Part model, mm, in its own coordinate system. A direction names the side the tool comes from. Coordinates: 2 decimals unless noted, no trailing zeros. Order: outer loops, then holes, each group sorted by start corner. A loop starts at its lowest first (then second) coordinate and runs counter-clockwise, first axis right, second up. Notation, with made-up numbers: M 52.25,-38.75 L 60.25,-38.75 A27 cw 60.25,0.25 Z; hole C 54.5,73 d10. An arc over 180 degrees is marked long. Write item = value, one per line. Start each with the question number.
from build123d import *

# Parameters (mm, degrees)
SKETCH_1_R          = 1.5
SKETCH_1_R_2        = 45
EXTRUDE_1_DEPTH     = 3
SKETCH_2_R          = 34
SKETCH_2_R_2        = 2
CUT_EXTRUDE_1_DEPTH = 157.95222203
SKETCH_3_W          = 10
SKETCH_3_H          = 3
EXTRUDE_2_DEPTH     = 2.5
SKETCH_5_R          = 0.75
CUT_EXTRUDE_2_DEPTH = 157.95222203
SKETCH_8_R          = 0.9
CUT_EXTRUDE_3_DEPTH = 157.95222203


with BuildPart() as part:
    # 草图1 → Extrude 1 (new body)
    with BuildSketch(Plane(origin=(0, 0, 0), x_dir=(1, 0, 0), z_dir=(0, 1, 0))):
        with BuildLine():
            Line((-60, 24.852813742), (-60, -24.852813742))
            Line((-60, -24.852813742), (-24.852813742, -60))
            Line((-24.852813742, -60), (24.852813742, -60))
            Line((24.852813742, -60), (60, -24.852813742))
            Line((60, -24.852813742), (60, 24.852813742))
            Line((60, 24.852813742), (60, 45.147186258))
            Line((60, 45.147186258), (44.671002135, 128.6127102))
            ThreePointArc((44.671002135, 128.6127102), (37.801285013, 140.366427757), (25, 145))
            Line((25, 145), (-25, 145))
            ThreePointArc((-25, 145), (-37.801285013, 140.366427757), (-44.671002135, 128.6127102))
            Line((-44.671002135, 128.6127102), (-60, 45.147186258))
            Line((-60, 45.147186258), (-60, 24.852813742))
        make_face()
        with Locations(Location((-6.35, 52, 0), (0, 0, 270))):
            Circle(SKETCH_1_R, mode=Mode.SUBTRACT)
        with Locations(Location((6.35, 52, 0), (0, 0, 270))):
            Circle(SKETCH_1_R, mode=Mode.SUBTRACT)
        with Locations(Location((6.35, -52, 0), (0, 0, 90))):
            Circle(SKETCH_1_R, mode=Mode.SUBTRACT)
        with Locations(Location((-6.35, -52, 0), (0, 0, 90))):
            Circle(SKETCH_1_R, mode=Mode.SUBTRACT)
        with Locations(Location((0, 0, 0), (0, 0, 270))):
            Circle(SKETCH_1_R_2, mode=Mode.SUBTRACT)
    extrude(amount=EXTRUDE_1_DEPTH)

    # 草图2 → 切除-拉伸1 (cut, through all)
    with BuildSketch(Plane(origin=(0, 3, 0), x_dir=(1, 0, 0), z_dir=(0, 1, 0))):
        with Locations(Location((0, 105, 0), (0, 0, 270))):
            Circle(SKETCH_2_R)
        with Locations(Location((-35, 52.5, 0), (0, 0, 270))):
            Circle(SKETCH_2_R_2)
        with Locations(Location((35, 52.5, 0), (0, 0, 270))):
            Circle(SKETCH_2_R_2)
        with Locations(Location((40.783850417, 124.017821778, 0), (0, 0, 270))):
            Circle(SKETCH_2_R_2)
        with Locations(Location((-40.783850417, 124.017821778, 0), (0, 0, 90))):
            Circle(SKETCH_2_R_2)
        with Locations(Location((-50, 40.147186258, 0), (0, 0, 270))):
            Circle(SKETCH_2_R_2)
        with Locations(Location((50, 40.147186258, 0), (0, 0, 90))):
            Circle(SKETCH_2_R_2)
        Polygon((28.087242696, 35.158310508), (35.158310508, 28.087242696), (44.547727215, 37.476659403), (37.476659403, 44.547727215), align=None)
        Polygon((-37.476659403, 44.547727215), (-44.547727215, 37.476659403), (-35.158310508, 28.087242696), (-28.087242696, 35.158310508), align=None)
    extrude(amount=-CUT_EXTRUDE_1_DEPTH, mode=Mode.SUBTRACT)

    # 草图3 → 凸台-拉伸2 (add)
    with BuildSketch(Plane.XY.offset(60)):
        with Locations((-12.5, 1.5)):
            Rectangle(SKETCH_3_W, SKETCH_3_H)
        with Locations((12.5, 1.5)):
            Rectangle(SKETCH_3_W, SKETCH_3_H)
    extrude(amount=EXTRUDE_2_DEPTH)

    # 草图5 → 切除-拉伸2 (cut, through all)
    with BuildSketch(Plane(origin=(0, 3, 0), x_dir=(1, 0, 0), z_dir=(0, 1, 0))):
        with Locations((-18.25, -60)):
            Circle(SKETCH_5_R)
        with Locations((-6.75, -60)):
            Circle(SKETCH_5_R)
        with Locations((6.75, -60)):
            Circle(SKETCH_5_R)
        with Locations((18.25, -60)):
            Circle(SKETCH_5_R)
        Polygon((-44.794179278, 105.501282313), (-40.264845988, 88.597580353), (-38.332994336, 89.115218444), (-42.862327625, 106.018920404), align=None)
        Polygon((42.862327625, 106.018920404), (38.332994336, 89.115218444), (40.264845988, 88.597580353), (44.794179278, 105.501282313), align=None)
        with BuildLine():
            Line((-60, 0), (-60, -24.852813742))
            Line((-60, -24.852813742), (-42.426406871, -42.426406871))
            ThreePointArc((-42.426406871, -42.426406871), (-55.432771951, -22.961005942), (-60, 0))
        make_face()
        with BuildLine():
            Line((60, -24.852813742), (42.426406871, -42.426406871))
            ThreePointArc((42.426406871, -42.426406871), (55.432771951, -22.961005942), (60, 0))
            Line((60, 0), (60, -24.852813742))
        make_face()
    extrude(amount=-CUT_EXTRUDE_2_DEPTH, mode=Mode.SUBTRACT)

    # 草图8 → 切除-拉伸3 (cut, through all)
    with BuildSketch(Plane(origin=(0, 3, 0), x_dir=(1, 0, 0), z_dir=(0, 1, 0))):
        with Locations((-44.561242137, 104.63194907)):
            Circle(SKETCH_8_R)
        with Locations((-42.629390484, 105.14958716)):
            Circle(SKETCH_8_R)
        with Locations((-38.565931476, 89.984551687)):
            Circle(SKETCH_8_R)
        with Locations((-40.497783129, 89.466913597)):
            Circle(SKETCH_8_R)
        with Locations((40.497783129, 89.466913597)):
            Circle(SKETCH_8_R)
        with Locations((38.565931476, 89.984551687)):
            Circle(SKETCH_8_R)
        with Locations((42.629390484, 105.14958716)):
            Circle(SKETCH_8_R)
        with Locations((44.561242137, 104.63194907)):
            Circle(SKETCH_8_R)
    extrude(amount=-CUT_EXTRUDE_3_DEPTH, mode=Mode.SUBTRACT)


solid = part.part
Item 1: Cut at A-A, the plane x = 0. Write the cut outline in (y, z), and give its area (3 significant figures).
Item 2: Cut at C-C, the plane z = -31.5. Write the cut outline in (x, y).
Item 3: Flat gauge pins, fed straight in: pin 1 (4 mm diameter, centred on x = -6.35, z = -52, fed in from -Y); pin 2 (1.2 mm diameter, centred on y = 2, z = 61.5, fed in from +X); pin 3 (0.9 mm diameter, centred on x = -21.5, y = 1, fed in from +Z); pin 4 (1.5 mm diameter, centred on x = -29, y = 1.5, fed in from -Z). Where does each tip first touch, or does it go through?
Item 4: Cut at B-B, the plane z = 21. Write the cut outline in (x, y), and give its area (3 significant figures).
Item 5: Wall check: line 1 along Z through (x, y) = (-18.5, 2.2); line 2 along Z through (x, y) = (-14, 0.7); line 3 along X through (y, z) = (1.95, -52.5). Give the ranges that are in metal, low to high. Write a range as [from, to].
Item 6: Pull direction X, two halves, no side cores. Call faces 1 (the cylindrical face through (38, 1.5, -140.2)), 2 (the flat face through (-52.23, 1.48, -87.46)), 3 (the cylindrical face through (33.048, 1.521, -52.934)): pulls with the +X half, pulls with the -X half, needs draft (parallel to the pull), parting line crosses it, or undercut.
Item 7: 3-axis set-ups, long thin cutter, end or side, ignore diameter. For faces 4 (the flat face through (39.79, 1.52, -32.72)), 5 (the flat face through (33.517, 1.479, 51.336)): which of +Z, -Z, +X, -X, +Y, -Y reach the whole face in a straight line?
Item 8: Cut at D-D, the plane y = 2.4. Count the separate pieces of the cut face and the enclosed holes in it, and give its area (3 significant figures).
Filled sheet:
q1.outline = M 0,-145 L 3,-145 L 3,-139 L 0,-139 Z; M 0,-71 L 3,-71 L 3,-45 L 0,-45 Z; M 0,45 L 3,45 L 3,60 L 0,60 Z
q1.area = 141 mm2
q2.outline = M -60,0 L -38.57,0 L -38.57,3 L -60,3 Z; M 38.57,0 L 60,0 L 60,3 L 38.57,3 Z
q3.pin_1 = 0
q3.pin_2 = 17.5
q3.pin_3 = 60
q3.pin_4 = -144.73
q4.outline = M -56.2,0 L -39.8,0 L -39.8,3 L -56.2,3 Z; M 39.8,0 L 56.2,0 L 56.2,3 L 39.8,3 Z
q4.area = 98.4 mm2
q5.line_1 = [-145, -133.53], [-76.47, -41.02], [41.02, 59.29]
q5.line_2 = [-145, -135.98], [-74.02, -42.77], [42.77, 62.5]
q5.line_3 = [-58.65, -37], [-33, -7.76], [-4.94, 4.94], [7.76, 33], [37, 58.65]
q6.face_1 = pulls with the +X half
q6.face_2 = pulls with the -X half
q6.face_3 = undercut
q7.face_4 = +Y, -Y
q7.face_5 = +Z, +X, +Y, -Y
q8.separate_pieces = 1
q8.enclosed_holes = 14
q8.area = 10,900 mm2
